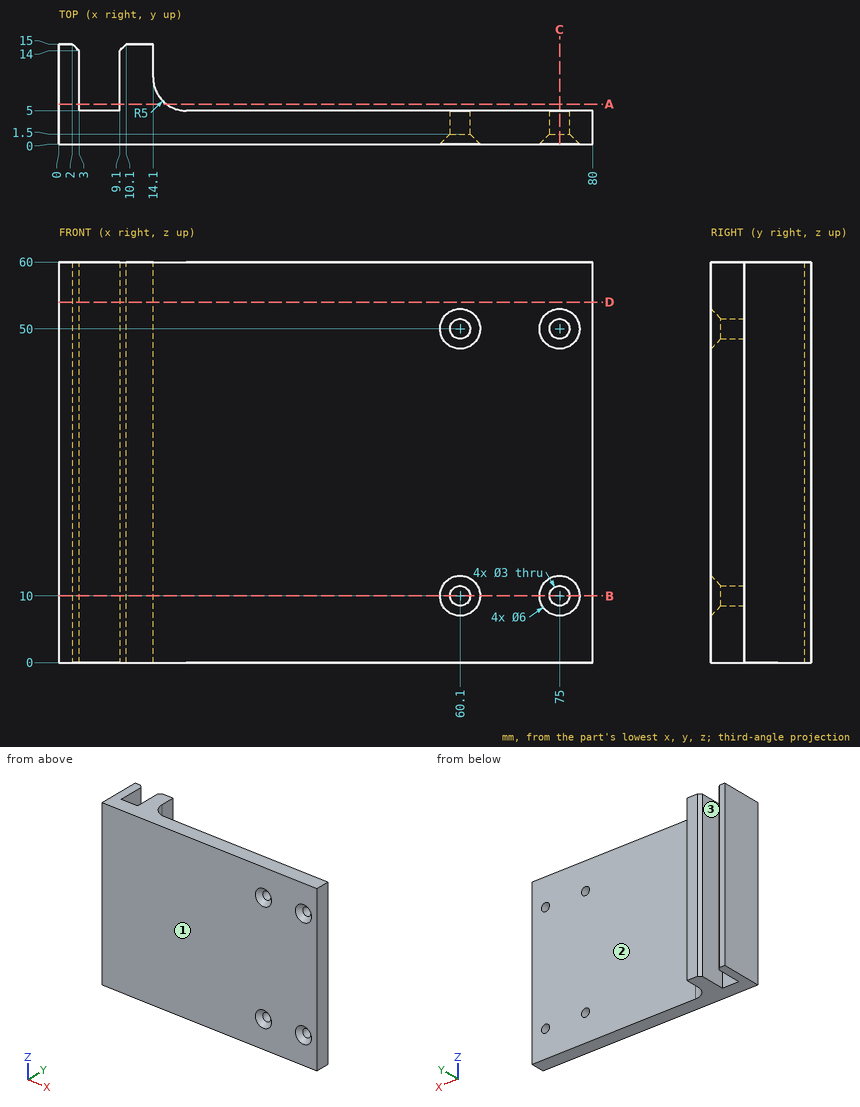
The drawing under review shows one solid part. Ordinate dimensions are in mm from its lowest x, y, z. A direction names the side the tool comes from. Coordinates: 2 decimals unless noted, no trailing zeros. Write each loop counter-clockwise with the first axis right and the second up, starting at its lowest first coordinate (ties: lowest second). Pieces come first, ordered by that corner, then holes.
1) Insertion check: pin 1 (1.5 mm diameter, centred on x = 60, z = 45, fed in from +Y); pin 2 (4 mm diameter, centred on x = 75, z = 10, fed in from -Y); pin 3 (4 mm diameter, centred on y = 4, z = 18, fed in from -X); pin 4 (1.5 mm diameter, centred on y = 13.5, z = 17.5, fed in from +X). Each pin has a flat end and moves straight along its axis. Give the tip position at first contact, or say it passes through.
2) Add section A-A (y = 6). Write out the cut boundary in (x, z), plus the area to 3 significant figures.
3) Add section B-B (z = 10). Write out the cut boundary in (x, y), plus the area to 3 significant figures.
4) Machinability: for the marked faces 1, 2 and 3, which of the approach directions +Z, -Z, +X, -X, +Y, -Y give a long, thin tool a straight path to every point of the face, cutting with its end or side? Answer none if there is none.
5) Add section C-C (x = 75). Write out the cut boundary in (y, z), plus the area to 4 significant figures.
6) Add section D-D (z = 54). Write out the cut boundary in (x, y), plus the area to 3 significant figures.
7) To check wall thickness, follow L1, parallel to Z at x = 75, y = 4; L2, parallel to X at y = 2.7, z = 10; L3, parallel to X at y = 13, z = 21.5. State the ranges of each line that lie inside material, in increasing order.
Check result:
1. pin 1: stops at y = 5
1. pin 2: stops at y = 1
1. pin 3: stops at x = 0
1. pin 4: stops at x = 14.1
2. outline: (0, 0) - (3, 0) - (3, 60) - (0, 60) - close; (9.1, 0) - (16.1, 0) - (16.1, 60) - (9.1, 60) - close
2. area: 600 mm2
3. outline: (0, 0) - (57.1, 0) - (58.6, 1.5) - (58.6, 5) - (19.1, 5) arc R5 cw to (14.1, 10) - (14.1, 15) - (10.1, 15) - (9.1, 14) - (9.1, 5) - (3, 5) - (3, 14) - (2, 15) - (0, 15) - close; (61.6, 1.5) - (63.1, 0) - (72, 0) - (73.5, 1.5) - (73.5, 5) - (61.6, 5) - close; (76.5, 1.5) - (78, 0) - (80, 0) - (80, 5) - (76.5, 5) - close
3. area: 450 mm2
4. face 1: +Z, -Z, +X, -X, -Y
4. face 2: +Z, -Z, +X, +Y
4. face 3: +Z, -Z, +Y
5. outline: (0, 0) - (5, 0) - (5, 8.5) - (1.5, 8.5) - (0, 7) - close; (0, 13) - (1.5, 11.5) - (5, 11.5) - (5, 48.5) - (1.5, 48.5) - (0, 47) - close; (0, 53) - (1.5, 51.5) - (5, 51.5) - (5, 60) - (0, 60) - close
5. area: 265.5 mm2
6. outline: (0, 0) - (80, 0) - (80, 5) - (19.1, 5) arc R5 cw to (14.1, 10) - (14.1, 15) - (10.1, 15) - (9.1, 14) - (9.1, 5) - (3, 5) - (3, 14) - (2, 15) - (0, 15) - close
6. area: 484 mm2
7. L1: z = 0 to 8.5, 11.5 to 48.5, 51.5 to 60
7. L2: x = 0 to 58.6, 61.6 to 73.5, 76.5 to 80
7. L3: x = 0 to 3, 9.1 to 14.1
